from build123d import *

# Parameters (mm, degrees)
BOX_W                     = 500
BOX_H                     = 500
BOX_DEPTH                 = 500
BOX_PLACEMENT_ANGLE       = 2
TUBE019_R                 = 85
TUBE019_R_2               = 80
TUBE019_DEPTH             = 21
TUBE012_R                 = 100
TUBE012_R_2               = 80
TUBE012_DEPTH             = 200
PAD030_DEPTH              = 100
PAD031_DEPTH              = 2
COMMON013_PLACEMENT_ANGLE = 45
ARRAY013_COUNT            = 22
ARRAY013_PLACEMENT_ANGLE  = 180
TUBE020_R                 = 34
TUBE020_R_2               = 30
TUBE020_DEPTH             = 21


with BuildPart() as cube:
    # Box → Box (new body)
    with BuildSketch(Plane.XY):
        with Locations((250, 250)):
            Rectangle(BOX_W, BOX_H)
    extrude(amount=BOX_DEPTH)


with BuildPart() as cube_1:
    # Box placement: moved
    add(cube.part.moved(Location((8.73, -250, 0))).rotate(Axis((8.73, -250, 0), (0, 0, 1)), BOX_PLACEMENT_ANGLE))


with BuildPart() as tube019:
    # Tube019 → Tube019 (new body)
    with BuildSketch(Plane.XY.offset(139.5)):
        Circle(TUBE019_R)
        Circle(TUBE019_R_2, mode=Mode.SUBTRACT)
    extrude(amount=TUBE019_DEPTH)


with BuildPart() as tube012:
    # Tube012 → Tube012 (new body)
    with BuildSketch(Plane.XY):
        Circle(TUBE012_R)
        Circle(TUBE012_R_2, mode=Mode.SUBTRACT)
    extrude(amount=TUBE012_DEPTH)


with BuildPart() as body031:
    # Sketch030 → Pad030 (new body)
    with BuildSketch(Plane.XZ):
        Polygon((0, 0), (0, 2), (26, 0.9), (26, 0), align=None)
    extrude(amount=PAD030_DEPTH)


with BuildPart() as body031_1:
    # Body031 placement: moved
    add(body031.part.moved(Location((-5, 0, 5))))


with BuildPart() as cut001:
    # Sketch031 → Pad031 (new body)
    with BuildSketch(Plane.XY):
        Polygon((0, 0), (0, -52), (25.94305, -47.924315), (8.5, 0), align=None)
    extrude(amount=PAD031_DEPTH)


with BuildPart() as cut001_1:
    # Body032 placement: moved
    add(cut001.part.moved(Location((-5, -33, 5))))

    # Common013: intersect Body031
    add(body031_1.part, mode=Mode.INTERSECT)


with BuildPart() as cut001_2:
    # Common013 placement: moved
    add(cut001_1.part.rotate(Axis((0, 0, 0), (0, 1, 0)), COMMON013_PLACEMENT_ANGLE))

    # Array013: Cut001 ×22 about axis
    array013_axis = Axis((0, 0, 0), (0, 0, 1))


with BuildPart() as cut001_3:
    add(cut001_2.part)
    for i in range(1, ARRAY013_COUNT):
        add(cut001_2.part.rotate(array013_axis, i * 360 / ARRAY013_COUNT))


with BuildPart() as cut001_4:
    # Array013 placement: moved
    add(cut001_3.part.moved(Location((0, 0, 149))).rotate(Axis((0, 0, 149), (0, 1, 0)), ARRAY013_PLACEMENT_ANGLE))

    # Cut001: cut Tube012
    add(tube012.part, mode=Mode.SUBTRACT)


with BuildPart() as obj1:
    # Tube020 → Tube020 (new body)
    with BuildSketch(Plane.XY.offset(139.5)):
        Circle(TUBE020_R)
        Circle(TUBE020_R_2, mode=Mode.SUBTRACT)
    extrude(amount=TUBE020_DEPTH)

    # Fusion009: union Tube019, Cut001
    add(tube019.part)
    add(cut001_4.part)

    # Common015: intersect Cube
    add(cube_1.part, mode=Mode.INTERSECT)


solid = obj1.part
Part model, mm, in its own coordinate system. A direction names the side the tool comes from. Coordinates: 2 decimals unless noted, no trailing zeros. Order: outer loops, then holes, each group sorted by start corner. A loop starts at its lowest first (then second) coordinate and runs counter-clockwise, first axis right, second up. Notation, with made-up numbers: (73.5, 48) - (79.5, 48) arc R20 ccw to (79.5, 85) - close; hole circle Ø1 at (60, 13). An arc over 180 degrees is marked (long way). Use CSV: the item, a comma, the result in double quotes.
Item 1: Drop flat-ended pins along their axis: P1, Ø12, axis at y = -3, z = 144, coming from the -X side; P2, Ø12, axis at y = -43.5, z = 154.5, coming from the +X side; P3, Ø2, axis at y = 1, z = 152.5, coming from the +X side. Give the stop position or say it passes through.
Solved:
P1,"stops at x = 28.62"
P2,"stops at x = 76.28"
P3,"stops at x = 85"
Item 2: Mould opens along Y. For faces 4 (the face through (84.993, 1.098, 149.853)), 5 (the face through (80, 7, 139.5)), 6 (the face through (23.796, 57.181, 148.651)) say: +Y half, -Y half, draft (parallel to the pull), parting line (faces both ways), or undercut.
Solved:
face 4,"parting line"
face 5,"draft"
face 6,"undercut"
Item 3: Probe probe 1 along X at (y, z) = (58, 151.5); probe 2 along X at (y, z) = (-66.5, 155.5) (3 decimals); probe 3 along Y at (x, z) = (71, 149). List the from-to ranges inside material, lowest first.
Solved:
probe 1,"x = 9.57 to 11.51, 27.01 to 29.02, 48.65 to 50.95, 55.1 to 62.14"
probe 2,"x = 4.009 to 5.382, 24.689 to 26.605, 44.472 to 52.941"
probe 3,"y = -46.73 to -36.86, -19.51 to -17.35, 0.9 to 3.06, 22.3 to 24.65, 36.86 to 46.73"
Item 4: 3-axis set-ups, long thin cutter, end or side, ignore diameter. For faces 1 (the face through (53.617, -20.194, 153.403)), 2 (the face through (24.84, 56.776, 147.506)), 3 (the face through (31, -2, 139.5)): which of +Z, -Z, +X, -X, +Y, -Y reach the whole face in a straight line?
Solved:
face 1,"+Z"
face 2,"-Z"
face 3,"-Z, +X, -X, +Y, -Y"
Item 5: Saw through at A-A on y = -41. Give the cut face in (x, z).
Solved:
outline,"(2.74, 148.69) - (10.56, 140.51) - (12.04, 141.93) - (3.79, 149.85) - close; (15.01, 149.36) - (24.67, 140.51) - (26.35, 141.93) - (16.09, 150.56) - close; (30.12, 151.23) - (45.16, 140.51) - (47.32, 141.93) - (31.27, 152.44) - close; (53.25, 155.49) - (68.69, 148.51) - (68.69, 139.5) - (74.46, 139.5) - (74.46, 160.5) - (68.69, 160.5) - (68.69, 150.69) - (54.49, 156.59) - close"
Item 6: Saw through at B-B on x = 50. Give the number of separate pieces and of enclosed holes in the cut face, and give its area (3 significant figures).
Solved:
separate pieces,"7"
enclosed holes,"0"
area,"478 mm²"
